Part model, mm, in its own coordinate system. Face numbers are marked on the shaded views. A direction names the side the tool comes from. Coordinates: 2 decimals unless noted, no trailing zeros. Write each loop counter-clockwise with the first axis right and the second up, starting at its lowest first coordinate (ties: lowest second). Pieces come first, ordered by that corner, then holes. Notation, with made-up numbers: (64.5, 0) - (90.5, 0) arc R36 cw to (90.5, 38) - close; hole circle Ø6 at (-22.75, -11). An arc over 180 degrees is marked (long way). Use one line per item in the form item = value. Start each with the question number.
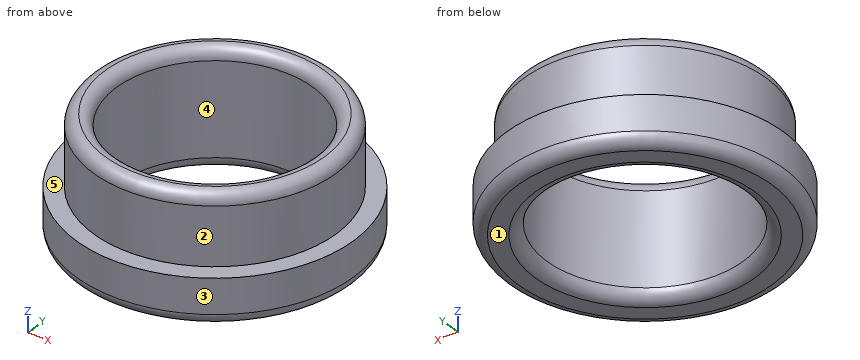
from build123d import *

# Parameters (mm, degrees)
F0_R     = 10.5
F0_R_2   = 8.5
F1_DEPTH = 10
F0_R_3   = 12
F2_DEPTH = 4
F3_R     = 0.99999


# Not quite as in the source:
# - a fillet or chamfer is up to 0.001 mm smaller than in the source, because OpenCascade refuses the exact size


with BuildPart() as f1:
    # F0 (on Top) → F1 (new body)
    with BuildSketch(Plane.XY):
        Circle(F0_R)
        Circle(F0_R_2, mode=Mode.SUBTRACT)
    extrude(amount=F1_DEPTH)

    # F0 (on Top) → F2 (join)
    with BuildSketch(Plane.XY):
        Circle(F0_R_3)
        Circle(F0_R, mode=Mode.SUBTRACT)
    extrude(amount=F2_DEPTH)

    # F3 (radius 1 in the source; OpenCascade refuses exactly that, so slightly less here)
    f3_edges = [f1.edges().sort_by_distance(p)[0] for p in [
        (-8.5, 0, 0),
        (-12, 0, 0),
        (-8.5, 0, 10),
        (-10.5, 0, 10),
    ]]
    fillet(f3_edges, radius=F3_R)


solid = f1.part
Q1. Which spindle directions (+Z, -Z, +X, -X, +Y, -Y) get a long thin tool onto all of the face, cutting with end or side? Do the marked faces 1 and 2. Say none if no direction does.
Q2. Drill centre lines: probe 1 along Y at (x, z) = (0, 4.5); probe 2 along Y at (x, z) = (0, 3.75); probe 3 along X at (y, z) = (-4.5, 1.25). Where is each one in solid material? Low to high.
Q3. Mould opens along X. For the marked faces 3, 4 and 5 say: released by +X, released by -X, zero draft, split by the parting line, or undercut.
Q4. Slice it at D-D (z = 1.75). List the corners of the cut face in (x, y).
Q5. Pin check, flat tips, straight feed: P1, Ø2, axis at y = 9.5, z = 6, coming from the -X side; P2, Ø2, axis at x = -8, y = -0.5, coming from the +Z side; P3, Ø2, axis at y = -8.5, z = 7.5, coming from the -X side. Stop position of each tip, or through.
Q6. Slice it at C-C (z = 5). List the corners of the cut face in (x, y), plus the area to 3 significant figures.
Solution:
q1.face_1 = -Z, +X, -X, +Y, -Y
q1.face_2 = +Z
q2.probe_1 = -10.5 to -8.5, 8.5 to 10.5
q2.probe_2 = -12 to -8.5, 8.5 to 12
q2.probe_3 = -11.12 to -7.21, 7.21 to 11.12
q3.face_3 = split by the parting line
q3.face_4 = undercut
q3.face_5 = zero draft
q4.outline = circle Ø24 at (0, 0); hole circle Ø17 at (0, 0)
q5.P1 = -6.16
q5.P2 = 9.87
q5.P3 = -7.35
q6.outline = circle Ø21 at (0, 0); hole circle Ø17 at (0, 0)
q6.area = 119 mm2
